Model file for the job. Use its own axes, mm. Round coordinates to 2 decimals unless told otherwise and drop trailing zeros. Order: outer loops, then holes, each group sorted by start corner. A loop starts at its lowest first (then second) coordinate and runs counter-clockwise, first axis right, second up. Notation, with made-up numbers: M -35,77.5 L -28,77.5 A10 ccw -28,84.5 Z; hole C 8,69.5 d2. An arc over 180 degrees is marked long. Return JSON: item names as keys, results as strings. Group by question number.
Item 1: Slice it at A-A on y = -0.75. Write the cut outline in (x, z), then the cut area to 3 significant figures.
Item 2: Probe line 1 along X through (y, z) = (0.7, -15.25); line 2 along X through (y, z) = (-0.1, 14.5); line 3 along Z through (x, y) = (49, -0.25). List the from-to ranges inside material, lowest first.
Item 3: Slice it at B-B on x = 64.5. Write the cut outline in (y, z).
Item 4: Pin check, flat tips, straight feed: pin 1 Ø0.9 at (x, y) = (66, 0) entering from +Z; pin 2 Ø4 at (x, z) = (-15.25, 15.25) entering from -Y. Stop position of each tip, or through.
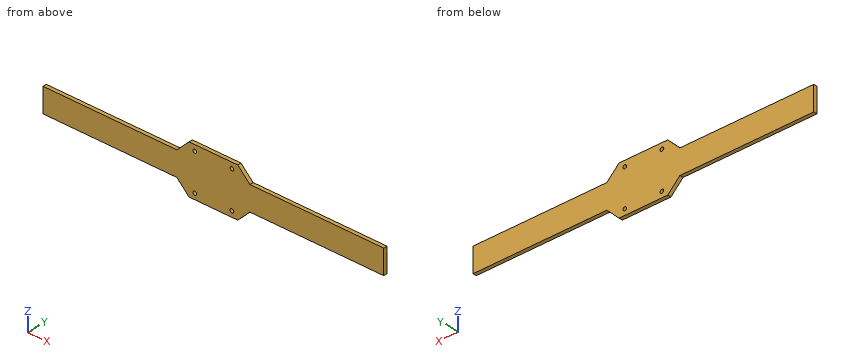
from build123d import *

# Parameters (mm, degrees)
SKETCH1_R           = 1.5
BOSS_EXTRUDE1_DEPTH = 1.5


with BuildPart() as part:
    # Sketch1 → Boss-Extrude1 (new, symmetric)
    with BuildSketch(Plane(origin=(0, 0, 0), x_dir=(1, 0, 0), z_dir=(0, 1, 0))):
        Polygon((30, 10), (20, 20), (-20, 20), (-30, 10), (-140, 10), (-140, -10), (-30, -10), (-20, -20), (20, -20), (30, -10), (140, -10), (140, 10), align=None)
        with Locations(Location((-15.25, -15.25, 0), (0, 0, 270))):
            Circle(SKETCH1_R, mode=Mode.SUBTRACT)
        with Locations(Location((15.25, -15.25, 0), (0, 0, 270))):
            Circle(SKETCH1_R, mode=Mode.SUBTRACT)
        with Locations(Location((-15.25, 15.25, 0), (0, 0, 270))):
            Circle(SKETCH1_R, mode=Mode.SUBTRACT)
        with Locations(Location((15.25, 15.25, 0), (0, 0, 270))):
            Circle(SKETCH1_R, mode=Mode.SUBTRACT)
    extrude(amount=BOSS_EXTRUDE1_DEPTH, both=True)


solid = part.part
Output values:
{
 "1": {"outline": "M -140,-10 L -30,-10 L -20,-20 L 20,-20 L 30,-10 L 140,-10 L 140,10 L 30,10 L 20,20 L -20,20 L -30,10 L -140,10 Z; hole C -15.25,-15.25 d3; hole C -15.25,15.25 d3; hole C 15.25,-15.25 d3; hole C 15.25,15.25 d3", "area": "6,570 mm²"},
 "2": {"line 1": "-24.75 to -16.75, -13.75 to 13.75, 16.75 to 24.75", "line 2": "-25.5 to -16.55, -13.95 to 13.95, 16.55 to 25.5", "line 3": "-10 to 10"},
 "3": {"outline": "M -1.5,-10 L 1.5,-10 L 1.5,10 L -1.5,10 Z"},
 "4": {"pin 1": "z = 10", "pin 2": "y = -1.5"}
}
